from build123d import *

# Parameters (mm, degrees)
F1_DEPTH  = 5.65
F2_R      = 2.25
F3_DEPTH  = 4
F4_R      = 3.875
F5_DEPTH  = 4.6
F7_DEPTH  = 5
F9_COUNT  = 10
F12_DEPTH = 4.6
F13_R     = 1.1


with BuildPart() as f1:
    # F0 (on Top) → F1 (new body)
    with BuildSketch(Plane.XY):
        Polygon((-0.5625, -0.974279), (0.5625, -0.974279), (1.125, 0), (0.5625, 0.974279), (-0.5625, 0.974279), (-1.125, 0), align=None)
    extrude(amount=F1_DEPTH)

    # F2 (on face) → F3 (join)
    with BuildSketch(Plane.XY.offset(5.65)):
        Circle(F2_R)
    extrude(amount=F3_DEPTH)

    # F4 (on face) → F5 (join)
    with BuildSketch(Plane.XY.offset(9.65)):
        Circle(F4_R)
    extrude(amount=F5_DEPTH)


with BuildPart() as f7:
    # F6 (on face) → F7 (new body)
    with BuildSketch(Plane.XY.offset(14.25)):
        with BuildLine():
            Line((3.842607, -0.5), (4.375, -0.5))
            Line((4.375, -0.5), (4.375, 0.5))
            Line((4.375, 0.5), (3.842607, 0.5))
            ThreePointArc((3.842607, 0.5), (3.866893, 0.250524), (3.875, 0))
            ThreePointArc((3.875, 0), (3.866893, -0.250524), (3.842607, -0.5))
        make_face()
        with BuildLine():
            Line((3.375, -0.5), (3.842607, -0.5))
            ThreePointArc((3.842607, -0.5), (3.866893, -0.250524), (3.875, 0))
            ThreePointArc((3.875, 0), (3.866893, 0.250524), (3.842607, 0.5))
            Line((3.842607, 0.5), (3.375, 0.5))
            Line((3.375, 0.5), (3.375, -0.5))
        make_face()
    extrude(amount=-F7_DEPTH)


with BuildPart() as f9_1:
    # F9: instance of F7
    add(f7.part.rotate(Axis((0, 0, 7.362194), (0, 0, -1)), 1 * 360 / F9_COUNT))


with BuildPart() as f9_2:
    # F9: instance of F7
    add(f7.part.rotate(Axis((0, 0, 7.362194), (0, 0, -1)), 2 * 360 / F9_COUNT))


with BuildPart() as f9_3:
    # F9: instance of F7
    add(f7.part.rotate(Axis((0, 0, 7.362194), (0, 0, -1)), 3 * 360 / F9_COUNT))


with BuildPart() as f9_4:
    # F9: instance of F7
    add(f7.part.rotate(Axis((0, 0, 7.362194), (0, 0, -1)), 4 * 360 / F9_COUNT))


with BuildPart() as f9_5:
    # F9: instance of F7
    add(f7.part.rotate(Axis((0, 0, 7.362194), (0, 0, -1)), 5 * 360 / F9_COUNT))


with BuildPart() as f9_6:
    # F9: instance of F7
    add(f7.part.rotate(Axis((0, 0, 7.362194), (0, 0, -1)), 6 * 360 / F9_COUNT))


with BuildPart() as f9_7:
    # F9: instance of F7
    add(f7.part.rotate(Axis((0, 0, 7.362194), (0, 0, -1)), 7 * 360 / F9_COUNT))


with BuildPart() as f9_8:
    # F9: instance of F7
    add(f7.part.rotate(Axis((0, 0, 7.362194), (0, 0, -1)), 8 * 360 / F9_COUNT))


with BuildPart() as f9_9:
    # F9: instance of F7
    add(f7.part.rotate(Axis((0, 0, 7.362194), (0, 0, -1)), 9 * 360 / F9_COUNT))


with BuildPart() as f1_1:
    add(f1.part)

    # F10: cut F7, F9_1, F9_2, F9_3, F9_4, F9_5, F9_6, F9_7, F9_8, F9_9
    add(f7.part, mode=Mode.SUBTRACT)
    add(f9_1.part, mode=Mode.SUBTRACT)
    add(f9_2.part, mode=Mode.SUBTRACT)
    add(f9_3.part, mode=Mode.SUBTRACT)
    add(f9_4.part, mode=Mode.SUBTRACT)
    add(f9_5.part, mode=Mode.SUBTRACT)
    add(f9_6.part, mode=Mode.SUBTRACT)
    add(f9_7.part, mode=Mode.SUBTRACT)
    add(f9_8.part, mode=Mode.SUBTRACT)
    add(f9_9.part, mode=Mode.SUBTRACT)

    # F11 (on face) → F12 (join)
    with BuildSketch(Plane.XY.offset(14.25)):
        with BuildLine():
            Line((-4.86289, -1), (-3.743745, -1))
            ThreePointArc((-3.743745, -1), (-3.801405, -0.751627), (-3.842607, -0.5))
            Line((-3.842607, -0.5), (-3.375, -0.5))
            Line((-3.375, -0.5), (-3.375, 0.5))
            Line((-3.375, 0.5), (-3.842607, 0.5))
            ThreePointArc((-3.842607, 0.5), (-3.801405, 0.751627), (-3.743745, 1))
            Line((-3.743745, 1), (-4.86289, 1))
            Line((-4.86289, 1), (-4.86289, -1))
        make_face()
    extrude(amount=-F12_DEPTH)

    # F13
    f13_edges = [f1_1.edges().sort_by_distance(p)[0] for p in [
        (-4.86289, 0, 14.25),
    ]]
    fillet(f13_edges, radius=F13_R)


solid = f1_1.part
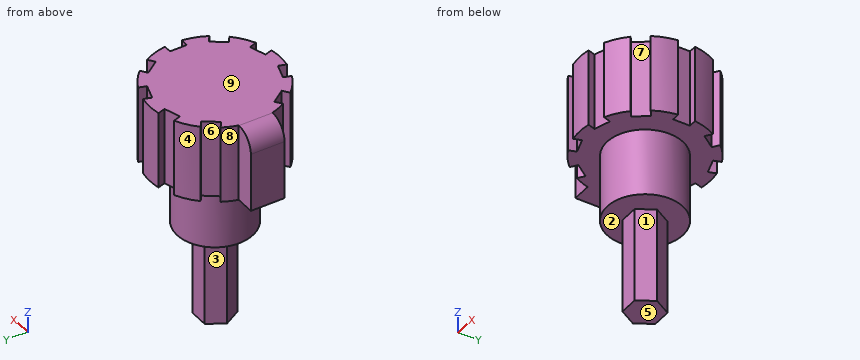
Geometry check sheet. Reference: the model listing, model coordinates, mm. Face numbers are marked on the shaded views. A direction names the side the tool comes from. Round coordinates to 2 decimals unless told otherwise and drop trailing zeros. Order: outer loops, then holes, each group sorted by start corner. A loop starts at its lowest first (then second) coordinate and runs counter-clockwise, first axis right, second up. Notation, with made-up numbers: M -38.75,47 L 17.25,47 A24 ccw 17.25,78 Z; hole C 35.25,58.5 d2. An arc over 180 degrees is marked long. Answer in a Markdown table with one row per item. Add a question column.
Item 1: Set-up check for the marked faces 1, 2, 3, 4 and 5: record each of +Z, -Z, +X, -X, +Y, -Y from which the full face is reachable in a straight line by a thin tool's end or side.
Item 2: Material ranges on L1, parallel to Y at x = 3.5, z = 9.75; L2, parallel to Z at x = -1, y = 0.75; L3, parallel to Y at x = -0.25, z = 1.75, recorded low to high. Write a range as [from, to].
Item 3: Sectioned sample at A-A, the plane x = 0. Enter the section's corners in (y, z) (3 decimals).
Item 4: Sectioned sample at D-D, the plane z = 9. Enter the section's corners in (x, y).
Item 5: Depth check by flat-ended pin: pin 1 Ø1 at (y, z) = (1, 8.5) entering from -X; pin 2 Ø0.5 at (y, z) = (0, 11.5) entering from +X (3 decimals); pin 3 Ø0.6 at (x, z) = (0, 2.5) entering from -Y. Enter the tip coordinate at first touch or a pass-through.
Item 6: Draft check along Y on the marked faces 6, 7, 8 and 9. Enter one of: released by +Y, released by -Y, zero draft, split by the parting line, or undercut.
Item 7: Sectioned sample at C-C, the plane y = 0.25. Enter the section's corners in (x, z) (3 decimals).
Item 8: Sectioned sample at B-B, the plane z = 5.5. Enter the section's corners in (x, y) (1 decimal).
Filled in:
| question | item | result |
|---|---|---|
| 1 | face 1 | -Z, +X, -Y |
| 1 | face 2 | -Z |
| 1 | face 3 | -Z, -X, +Y |
| 1 | face 4 | +Z, -Z, -X, +Y |
| 1 | face 5 | -Z, +X, -X, +Y, -Y |
| 2 | L1 | y = [-1.66, -0.5], [0.5, 1.66] |
| 2 | L2 | z = [5.65, 14.25] |
| 2 | L3 | y = [-0.97, 0.97] |
| 3 | outline | M -3.875,9.65 L -2.25,9.65 L -2.25,5.65 L -0.974,5.65 L -0.974,0 L 0.974,0 L 0.974,5.65 L 2.25,5.65 L 2.25,9.65 L 3.875,9.65 L 3.875,14.25 L -3.875,14.25 Z |
| 4 | outline | C 0,0 d4.5 |
| 5 | pin 1 | stops at x = -2.19 |
| 5 | pin 2 | stops at x = 3.375 |
| 5 | pin 3 | stops at y = -0.97 |
| 6 | face 6 | undercut |
| 6 | face 7 | undercut |
| 6 | face 8 | released by +Y |
| 6 | face 9 | zero draft |
| 7 | outline | M -4.863,9.65 L -2.236,9.65 L -2.236,5.65 L -0.981,5.65 L -0.981,0 L 0.981,0 L 0.981,5.65 L 2.236,5.65 L 2.236,9.65 L 3.375,9.65 L 3.375,14.25 L -3.763,14.25 A1.1 ccw -4.863,13.15 Z |
| 8 | outline | M -1.1,0 L -0.6,-1 L 0.6,-1 L 1.1,0 L 0.6,1 L -0.6,1 Z |
